```python
from build123d import *


with BuildPart() as part:
    # CopySketch002 → AdditiveLoft section 0
    with BuildSketch(Plane.XY.offset(14.8)):
        Polygon((-10.399994, -3.3), (-6.399994, -3.3), (-6.399994, -1), (6.399994, -1), (6.399994, -3.3), (10.399994, -3.3), (10.400006, -1.7), (8.400006, -1.7), (8.400006, 1.7), (10.400006, 1.7), (10.400006, 3.3), (6.400006, 3.3), (6.400006, 1), (-6.399994, 1), (-6.399994, 3.3), (-10.399994, 3.3), (-10.399994, 1.7), (-8.399994, 1.7), (-8.399994, -1.7), (-10.399994, -1.7), align=None)
    # Sketch001 (on Plane) → AdditiveLoft section 1
    with BuildSketch(Plane.XY):
        Polygon((-14.899994, -3.3), (-10.899994, -3.3), (-10.899994, -1), (10.899994, -1), (10.899994, -3.3), (14.899994, -3.3), (14.900006, -1.7), (12.900006, -1.7), (12.900006, 1.7), (14.900006, 1.7), (14.900006, 3.3), (10.900006, 3.3), (10.900006, 1), (-10.899994, 1), (-10.899994, 3.3), (-14.899994, 3.3), (-14.899994, 1.7), (-12.899994, 1.7), (-12.899994, -1.7), (-14.899994, -1.7), align=None)
    loft()


solid = part.part
```
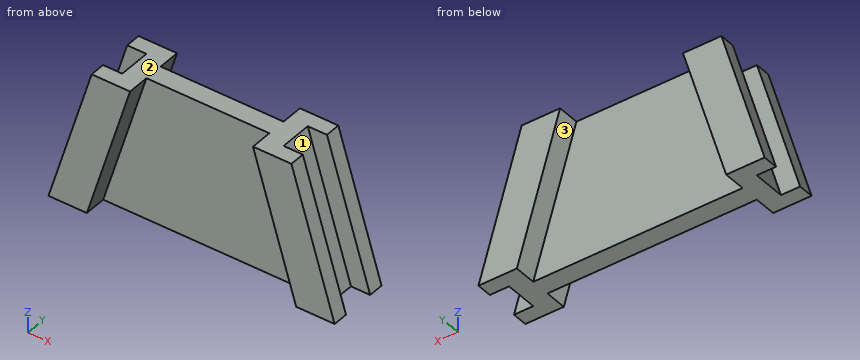
Design review of the part built by this model. Coordinates are the model's own, in mm. Face numbers are marked on the shaded views. Coordinates: 2 decimals unless noted, no trailing zeros. Order: outer loops, then holes, each group sorted by start corner. A loop starts at its lowest first (then second) coordinate and runs counter-clockwise, first axis right, second up.
1) Take a section at A-A, the plane y = 0. Give the boundary of the cut face in (x, z), and give its area (3 significant figures).
2) Mouldability with a two-part tool opening along X and no side actions: class the marked faces 1, 2 and 3 as +X half, -X half, draft (parallel to the pull), parting line (faces both ways), or undercut.
3) Wall thickness on line 1 along Y through (x, z) = (-11.5, 7.5); line 2 along Y through (x, z) = (7, 6); line 3 along X through (y, z) = (-2.5, 11): over which ranges is each line inside the solid? List them lowest first.
4) Clearance check with flat-ended pins moving along their axes: pin 1 (3 mm diameter, centred on x = -0.5, z = 10, fed in from +Y); pin 2 (3 mm diameter, centred on x = -7, z = 4.5, fed in from -Y); pin 3 (2 mm diameter, centred on y = -2, z = 11.5, fed in from -X). State where each tip first meets the part, or that it passes through.
Returned:
1. outline: (-12.9, 0) - (12.9, 0) - (8.4, 14.8) - (-8.4, 14.8) - close
1. area: 315 mm2
2. face 1: +X half
2. face 2: draft
2. face 3: undercut
3. line 1: y = -3.3 to -1.7, 1.7 to 3.3
3. line 2: y = -1 to 1
3. line 3: x = -11.56 to -7.56, 7.56 to 11.56
4. pin 1: stops at y = 1
4. pin 2: stops at y = -1
4. pin 3: stops at x = -11.71
